Model file for the job. Use its own axes, mm. Face numbers are marked on the shaded views. A direction names the side the tool comes from. Round coordinates to 2 decimals unless told otherwise and drop trailing zeros. Loops run counter-clockwise (first coordinate to the right, second up) from the corner with the lowest first, then second, coordinate; pieces in that order, holes last.
from build123d import *

# Parameters (mm, degrees)
SKETCH1_R           = 2
BOSS_EXTRUDE1_DEPTH = 4.1
SKETCH2_R           = 1.5
BOSS_EXTRUDE2_DEPTH = 7.9
CHAMFER1_SIZE       = 0.2


with BuildPart() as part:
    # Sketch1 → Boss-Extrude1 (new body)
    with BuildSketch(Plane(origin=(0, 0, 0), x_dir=(0, 0, -1), z_dir=(1, 0, 0))):
        Circle(SKETCH1_R)
    extrude(amount=BOSS_EXTRUDE1_DEPTH)

    # Sketch2 → Boss-Extrude2 (add)
    with BuildSketch(Plane.ZY):
        with Locations(Location((0, 0, 0), (0, 0, 180))):
            Circle(SKETCH2_R)
    extrude(amount=BOSS_EXTRUDE2_DEPTH)

    # Chamfer1
    chamfer1_edges = [part.edges().sort_by_distance(p)[0] for p in [
        (-7.9, 0, 1.5),
    ]]
    chamfer(chamfer1_edges, length=CHAMFER1_SIZE)


solid = part.part
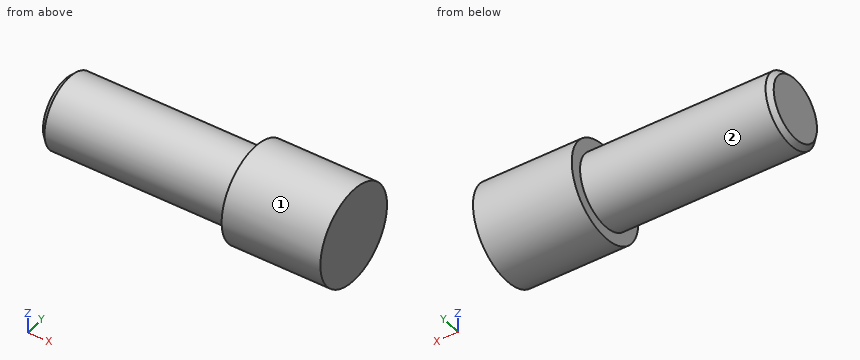
Q1. Slice it at C-C on x = 0.5. Give the cut face in (y, z), plus the area to 3 significant figures.
Q2. Tool access for the marked faces 1 and 2: list every direction of +Z, -Z, +X, -X, +Y, -Y with a clear straight run to the whole face (end or side of a thin tool).
Q3. Slice it at A-A on y = 0. Give the cut face in (x, z), plus the area to 3 significant figures.
Q4. Flat gauge pins, fed straight in: P1, Ø1.5, axis at x = -3.5, y = -1, coming from the -Z side; P2, Ø1.5, axis at x = -2, z = -1, coming from the -Y side; P3, Ø1.5, axis at x = -5.5, y = 1, coming from the +Z side. Where does each tip first touch, or does it go through?
Q5. Slice it at D-D on x = -5.25. Give the cut face in (y, z).
Q6. Probe line 1 (X direction, y = 1.2, z = -1.35); line 2 (Y direction, x = 1, z = -0.1); line 3 (Y direction, x = -5.75, z = -0.5). List the from-to ranges inside material, lowest first.
Reply:
1. outline: circle Ø4 at (0, 0)
1. area: 12.6 mm2
2. face 1: +X, -X
2. face 2: -X
3. outline: (-7.9, -1.3) - (-7.7, -1.5) - (0, -1.5) - (0, -2) - (4.1, -2) - (4.1, 2) - (0, 2) - (0, 1.5) - (-7.7, 1.5) - (-7.9, 1.3) - close
3. area: 40.1 mm2
4. P1: stops at z = -1.48
4. P2: stops at y = -1.48
4. P3: stops at z = 1.48
5. outline: circle Ø3 at (0, 0)
6. line 1: x = 0 to 4.1
6. line 2: y = -2 to 2
6. line 3: y = -1.41 to 1.41
